from build123d import *

# Parameters (mm, degrees)
F0_W     = 508
F0_H     = 127
F1_DEPTH = 12.7
F3_D     = 3.175
F5_D     = 3.175
F7_D     = 76.2
F9_D     = 50.8
F11_D    = 76.2


with BuildPart() as f1:
    # F0 (on Front) → F1 (new body)
    with BuildSketch(Plane.XZ):
        with Locations((-143.865749, 51.691295)):
            Rectangle(F0_W, F0_H)
    extrude(amount=F1_DEPTH)

    # F3 (through all)
    with Locations(Plane.XZ.offset(12.7)):
        with Locations((100.726366, 106.68204)):
            Hole(F3_D / 2)

    # F5 (through all)
    with Locations(Plane.XZ.offset(12.7)):
        with Locations((101.377115, -4.356061), (-389.453292, 106.042355), (-389.003724, -4.472178)):
            Hole(F5_D / 2)

    # F7 (through all)
    with Locations(Plane.XZ.offset(12.7)):
        with Locations((-340.738475, 51.691294)):
            Hole(F7_D / 2)

    # F9 (through all)
    with Locations(Plane.XZ.offset(12.7)):
        with Locations((-73.235735, 53.365439)):
            Hole(F9_D / 2)

    # F11 (through all)
    with Locations(Plane.XZ.offset(12.7)):
        with Locations((54.064672, 51.691295)):
            Hole(F11_D / 2)


solid = f1.part
Model file for the job. Use its own axes, mm. Round coordinates to 2 decimals unless told otherwise and drop trailing zeros. Loops run counter-clockwise (first coordinate to the right, second up) from the corner with the lowest first, then second, coordinate; pieces in that order, holes last. Notation, with made-up numbers: (-7.5, -8) -> (2.5, -8) arc R23 ccw to (2.5, 26) -> close; hole circle Ø10 at (78.5, 85.5). An arc over 180 degrees is marked (long way). Answer as CSV lines item,"result". Start each with the question number.
1) Slice it at B-B (y = -8.25). List the corners of the cut face in (x, z) (1 decimal).
2) Mould opens along Z. For faces 1 (the face through (-147, 0, 53)), 2 (the face through (-147, -6, -11.809)), 3 (the face through (-97.463, -6.261, 60.995)) say: +Z half, -Z half, draft (parallel to the pull), parting line (faces both ways), or undercut.
3) Slice it at C-C (z = 71). List the corners of the cut face in (x, y).
4) Slice it at A-A (x = 38.5). List the corners of the cut face in (y, z).
5) Pin check, flat tip, straight feed: P1, Ø3, axis at x = -389.45, z = 106.04, coming from the +Y side. Stop position of the tip, or through.
6) Probe line 1 along X through (y, z) = (-1.25, 52.5); line 2 along X through (y, z) = (-5.25, 83); line 3 along X through (y, z) = (-0.75, -3.5). List the from-to ranges inside material, lowest first.
7) Slice it at D-D (x = -319). List the corners of the cut face in (y, z), plus the area to 3 significant figures.
Filled in:
1,outline,"(-397.9, -11.8) -> (110.1, -11.8) -> (110.1, 115.2) -> (-397.9, 115.2) -> close; hole circle Ø3.2 at (-389.5, 106); hole circle Ø3.2 at (-389, -4.5); hole circle Ø76.2 at (-340.7, 51.7); hole circle Ø50.8 at (-73.2, 53.4); hole circle Ø76.2 at (54.1, 51.7); hole circle Ø3.2 at (100.7, 106.7); hole circle Ø3.2 at (101.4, -4.4)"
2,face 1,"draft"
2,face 2,"-Z half"
2,face 3,"undercut"
3,outline,"(-397.87, -12.7) -> (-373.58, -12.7) -> (-373.58, 0) -> (-397.87, 0) -> close; (-307.89, -12.7) -> (-91.52, -12.7) -> (-91.52, 0) -> (-307.89, 0) -> close; (-54.96, -12.7) -> (21.22, -12.7) -> (21.22, 0) -> (-54.96, 0) -> close; (86.91, -12.7) -> (110.13, -12.7) -> (110.13, 0) -> (86.91, 0) -> close"
4,outline,"(-12.7, -11.81) -> (0, -11.81) -> (0, 16.92) -> (-12.7, 16.92) -> close; (-12.7, 86.47) -> (0, 86.47) -> (0, 115.19) -> (-12.7, 115.19) -> close"
5,P1,"passes through"
6,line 1,"x = -397.87 to -378.83, -302.65 to -98.62, -47.85 to 15.97, 92.16 to 110.13"
6,line 2,"x = -397.87 to -362.45, -319.03 to 32.35, 75.78 to 110.13"
6,line 3,"x = -397.87 to -390.26, -387.75 to 100.04, 102.71 to 110.13"
7,outline,"(-12.7, -11.81) -> (0, -11.81) -> (0, 20.4) -> (-12.7, 20.4) -> close; (-12.7, 82.98) -> (0, 82.98) -> (0, 115.19) -> (-12.7, 115.19) -> close"
7,area,"818 mm2"
